from build123d import *

# Parameters (mm, degrees)
SKETCH1_R           = 22
BOSS_EXTRUDE1_DEPTH = 8
SKETCH2_R           = 16.5
BOSS_EXTRUDE2_DEPTH = 0.5
SKETCH3_R           = 15.125
BOSS_EXTRUDE3_DEPTH = 6.8
SKETCH4_R           = 6
CUT_EXTRUDE1_DEPTH  = 35.671169579
SKETCH5_R           = 1.6
CUT_EXTRUDE2_DEPTH  = 7
CIRPATTERN1_COUNT   = 6
SKETCH6_R           = 2.2
CUT_EXTRUDE3_DEPTH  = 5.5
CIRPATTERN2_COUNT   = 4


with BuildPart() as part:
    # Sketch1 → Boss-Extrude1 (new body)
    with BuildSketch(Plane(origin=(0, 0, 0), x_dir=(1, 0, 0), z_dir=(0, 1, 0))):
        with Locations(Location((0, 0, 0), (0, 0, 270))):
            Circle(SKETCH1_R)
    extrude(amount=BOSS_EXTRUDE1_DEPTH)

    # Sketch2 → Boss-Extrude2 (add)
    with BuildSketch(Plane(origin=(0, 8, 0), x_dir=(1, 0, 0), z_dir=(0, 1, 0))):
        with Locations(Location((0, 0, 0), (0, 0, 270))):
            Circle(SKETCH2_R)
    extrude(amount=BOSS_EXTRUDE2_DEPTH)

    # Sketch3 → Boss-Extrude3 (add)
    with BuildSketch(Plane(origin=(0, 8.5, 0), x_dir=(1, 0, 0), z_dir=(0, 1, 0))):
        with Locations(Location((0, 0, 0), (0, 0, 270))):
            Circle(SKETCH3_R)
    extrude(amount=BOSS_EXTRUDE3_DEPTH)

    # Sketch4 → Cut-Extrude1 (cut, through all)
    with BuildSketch(Plane(origin=(0, 15.3, 0), x_dir=(1, 0, 0), z_dir=(0, 1, 0))):
        with Locations(Location((0, 0, 0), (0, 0, 270))):
            Circle(SKETCH4_R)
    extrude(amount=-CUT_EXTRUDE1_DEPTH, mode=Mode.SUBTRACT)

    # Sketch5 → Cut-Extrude2 (cut)
    with BuildSketch(Plane(origin=(0, 0, 0), x_dir=(1, 0, 0), z_dir=(0, 1, 0))):
        with Locations(Location((18.272234301, 2.894037603, 0), (0, 0, 270))):
            Circle(SKETCH5_R)
    cut_extrude2 = extrude(amount=CUT_EXTRUDE2_DEPTH, mode=Mode.SUBTRACT)

    # CirPattern1: Cut-Extrude2 ×6 about axis
    cirpattern1_axis = Axis((0, 0, 0), (0, 1, 0))
    for i in range(1, CIRPATTERN1_COUNT):
        add(cut_extrude2.rotate(cirpattern1_axis, i * 360 / CIRPATTERN1_COUNT), mode=Mode.SUBTRACT)

    # Sketch6 → Cut-Extrude3 (cut)
    with BuildSketch(Plane(origin=(0, 15.3, 0), x_dir=(1, 0, 0), z_dir=(0, 1, 0))):
        with Locations(Location((10.5, 0, 0), (0, 0, 270))):
            Circle(SKETCH6_R)
    cut_extrude3 = extrude(amount=-CUT_EXTRUDE3_DEPTH, mode=Mode.SUBTRACT)

    # CirPattern2: Cut-Extrude3 ×4 about axis
    cirpattern2_axis = Axis((0, 0, 0), (0, 1, 0))
    for i in range(1, CIRPATTERN2_COUNT):
        add(cut_extrude3.rotate(cirpattern2_axis, i * 360 / CIRPATTERN2_COUNT), mode=Mode.SUBTRACT)


solid = part.part
Here's how the part is built. I have some questions about the finished solid (model axes, mm). A direction names the side the tool comes from. Coordinates: 2 decimals unless noted, no trailing zeros. Write each loop counter-clockwise with the first axis right and the second up, starting at its lowest first coordinate (ties: lowest second). Pieces come first, ordered by that corner, then holes.
Item 1: On a 3-axis mill with a long thin cutter (end or side, diameter ignored), from which of +Z, -Z, +X, -X, +Y, -Y can I reach the whole of each face in a straight line? I mean faces 1 (the cylindrical face through (19.86, 3.45, -3.1)), 2 (the cylindrical face through (1.802, 7.757, 5.723)), 3 (the cylindrical face through (12.355, 12.588, 1.183)). Say none if no direction works.
Item 2: I want a section at A-A on z = 0. Write out the boundary of the cut face in (x, y) (3 decimals).
Item 3: Will these pins go through, and if not, where does the flat tip stop? pin 1 (6 mm diameter, centred on x = 8, y = 10.5, fed in from -Z); pin 2 (2 mm diameter, centred on x = 0, z = 11, fed in from +Y); pin 3 (4 mm diameter, centred on y = 8, z = -7, fed in from +X).
Item 4: I want a section at C-C on x = -3. Write out the boundary of the cut face in (y, z).
Item 5: If we mould it in two halves opening along X, with no side actions, what happens to faces 4 (the cylindrical face through (-14.765, 11.852, -3.279)), 5 (the cylindrical face through (-19.86, 3.45, 3.1)), 6 (the flat face through (16.4, 8, 3.2)), 7 (the cylindrical face through (-12.26, 3.45, -12.9))? For each: +X half, -X half, draft (parallel to the pull), parting line (faces both ways), or undercut.
Item 6: If I drill on line 1 (X direction, y = 11.2, z = 0) (3 decimals); line 2 (X direction, y = 1, z = 4); line 3 (Y direction, x = -6, z = 18), over which ranges is the centre line in solid material (lowest first)?
Item 7: I want a section at D-D on y = 2.5. Write out the boundary of the cut face in (x, z).
Item 8: I want a section at B-B on y = 13.5. Write out the boundary of the cut face in (x, z) (3 decimals).
Findings below:
1. face 1: -Y
1. face 2: +Y, -Y
1. face 3: +Y
2. outline: (-22, 0) - (-6, 0) - (-6, 15.3) - (-8.3, 15.3) - (-8.3, 9.8) - (-12.7, 9.8) - (-12.7, 15.3) - (-15.125, 15.3) - (-15.125, 8.5) - (-16.5, 8.5) - (-16.5, 8) - (-22, 8) - close; (6, 0) - (22, 0) - (22, 8) - (16.5, 8) - (16.5, 8.5) - (15.125, 8.5) - (15.125, 15.3) - (12.7, 15.3) - (12.7, 9.8) - (8.3, 9.8) - (8.3, 15.3) - (6, 15.3) - close
3. pin 1: stops at z = -21.07
3. pin 2: stops at y = 9.8
3. pin 3: stops at x = 21.42
4. outline: (0, -21.79) - (8, -21.79) - (8, -16.22) - (8.5, -16.22) - (8.5, -14.82) - (15.3, -14.82) - (15.3, -5.2) - (0, -5.2) - close; (0, 5.2) - (15.3, 5.2) - (15.3, 14.82) - (8.5, 14.82) - (8.5, 16.22) - (8, 16.22) - (8, 21.79) - (0, 21.79) - close
5. face 4: parting line
5. face 5: undercut
5. face 6: draft
5. face 7: undercut
6. line 1: x = -15.125 to -12.7, -8.3 to -6, 6 to 8.3, 12.7 to 15.125
6. line 2: x = -21.63 to -19.43, -17.12 to -4.47, 4.47 to 21.63
6. line 3: y = 7 to 8
7. outline: circle Ø44 at (0, 0); hole circle Ø3.2 at (-18.27, 2.89); hole circle Ø3.2 at (-11.64, -14.38); hole circle Ø3.2 at (-6.63, 17.27); hole circle Ø12 at (0, 0); hole circle Ø3.2 at (6.63, -17.27); hole circle Ø3.2 at (11.64, 14.38); hole circle Ø3.2 at (18.27, -2.89)
8. outline: circle Ø30.25 at (0, 0); hole circle Ø4.4 at (-10.5, 0); hole circle Ø12 at (0, 0); hole circle Ø4.4 at (0, -10.5); hole circle Ø4.4 at (0, 10.5); hole circle Ø4.4 at (10.5, 0)
